Source: CAD feature listing. Evaluate the final solid. Frame: model axes, mm. Give positions to 0.01 mm unless a question says otherwise; leave off trailing zeros. Loops run counter-clockwise (first coordinate to the right, second up) from the corner with the lowest first, then second, coordinate; pieces in that order, holes last. Notation, with made-up numbers: (31.25, -20) -> (54.25, -20) arc R15 ccw to (54.25, -1) -> close; hole circle Ø5 at (-22, -25). An arc over 180 degrees is marked (long way). Put each result on its own line as item: value.
Autodesk Inventor part; units mm, degrees
ref_plane "YZ Plane" through (0, 0, 0) normal (1, 0, 0) x (0, 1, 0)
ref_plane "XZ Plane" through (0, 0, 0) normal (0, 1, 0) x (-1, 0, 0)
ref_plane "XY Plane" through (0, 0, 0) normal (0, 0, 1) x (1, 0, 0)
sketch "Sketch2" plane through (0, 0, 0) normal (0, 1, 0) x (-1, 0, 0)
  line L0 (-179.5, 499.25) -> (179.5, 499.25)
  line L1 (179.5, 499.25) -> (179.5, -499.25)
  line L2 (179.5, -499.25) -> (-179.5, -499.25)
  line L3 (-179.5, -499.25) -> (-179.5, 499.25)
  line L4 (-179.5, 499.25) -> (179.5, -499.25) construction
  line L5 (179.5, 499.25) -> (-179.5, -499.25) construction
  point P0 (0, 0)
  dimension "d2" = 359
  dimension "d3" = 998.5
extrude "Plate1" add sketch "Sketch2" along normal blind 0.5
sketch "Sketch3" plane through (-179, 0.5, -499.25) normal (-1, 0, 0) x (0, -1, 0)
  line L0 (0, 998.5) -> (0, 0)
  line L1 (0, 0) -> (50, 0)
  line L2 (50, 0) -> (50, 998.5)
  line L3 (50, 998.5) -> (0, 998.5)
edge flange "Flange1" height 50 angle 90 thickness 0.5 bend radius 0.5 thickness toward (-1, 0, 0) relief tear relief width 0.5 relief depth 0.25 edges at (-179.5, 0, 0) wall of the first edge with corners at (-179, 0.5, 499.25) (-179, 0.5, -499.25) (-179, -49.5, -499.25) (-179, -49.5, 499.25)
bend "Bend1"
corner "Corner1"
sketch "Sketch6" plane through (179, 0.5, 499.25) normal (1, 0, 0) x (0, 1, 0)
  line L0 (0, -998.5) -> (0, 0)
  line L1 (0, 0) -> (-10, 0)
  line L2 (-10, 0) -> (-10, -998.5)
  line L3 (-10, -998.5) -> (0, -998.5)
edge flange "Flange4" height 10 angle 90 thickness 0.5 bend radius 0.5 thickness toward (1, 0, 0) relief tear relief width 0.5 relief depth 0.25 edges at (179.5, 0, 0) wall of the first edge with corners at (179, 0.5, -499.25) (179, 0.5, 499.25) (179, -9.5, 499.25) (179, -9.5, -499.25)
bend "Bend4"
corner "Corner4"
sketch "Sketch7" plane through (179.5, -9, 499.25) normal (0, -1, 0) x (1, 0, 0)
  line L0 (0, -998.5) -> (0, 0)
  line L1 (0, 0) -> (-10, 0)
  line L2 (-10, 0) -> (-10, -998.5)
  line L3 (-10, -998.5) -> (0, -998.5)
edge flange "Flange5" height 10 angle 90 thickness 0.5 bend radius 0.5 thickness toward (0, -1, 0) relief tear relief width 0.5 relief depth 0.25 edges at (179, -9.5, 0) wall of the first edge with corners at (179.5, -9, -499.25) (179.5, -9, 499.25) (169.5, -9, 499.25) (169.5, -9, -499.25)
bend "Bend5"
corner "Corner5"
equation "\"d3\" = Ancho - 3 * Thickness"
equation "\"d4\" = Thickness"
equation "\"d5\" = BendReliefWidth"
equation "\"d6\" = BendReliefDepth"
equation "\"d7\" = MinimumRemnant"
equation "\"d8\" = TransitionRadius"
equation "\"d11\" = BendRadius"
equation "\"d12\" = CornerReliefSize"
equation "\"d13\" = GapSize"
equation "\"d14\" = JacobiRadiusSize"
equation "\"d35\" = BendReliefWidth"
equation "\"d36\" = BendReliefDepth"
equation "\"d37\" = MinimumRemnant"
equation "\"d38\" = TransitionRadius"
equation "\"d41\" = BendRadius"
equation "\"d42\" = CornerReliefSize"
equation "\"d43\" = GapSize"
equation "\"d44\" = JacobiRadiusSize"
equation "\"d45\" = BendReliefWidth"
equation "\"d46\" = BendReliefDepth"
equation "\"d47\" = MinimumRemnant"
equation "\"d48\" = TransitionRadius"
equation "\"d51\" = BendRadius"
equation "\"d52\" = CornerReliefSize"
equation "\"d53\" = GapSize"
equation "\"d54\" = JacobiRadiusSize"
equation "\"BendRadius\" = Thickness"
equation "\"BendReliefWidth\" = Thickness"
equation "\"BendReliefDepth\" = 0.5 * Thickness"
equation "\"CornerReliefSize\" = 4 * Thickness"
equation "\"MinimumRemnant\" = 2 * Thickness"
equation "\"TransitionRadius\" = BendRadius"
equation "\"JacobiRadiusSize\" = BendRadius"
equation "\"GapSize\" = Thickness"
equation "\"Space5\" = 0"
equation "\"Space6\" = 0"
equation "\"Space7\" = 0"
properties part number "Divisor"
(1) Section A-A on z = 436. Return loops of the section in (x, y).
Calculated:
outline: (-179.5, -49.5) -> (-179, -49.5) -> (-179, -0.5) arc R0.5 cw to (-178.5, 0) -> (178.5, 0) arc R0.5 cw to (179, -0.5) -> (179, -8.5) arc R0.5 cw to (178.5, -9) -> (169.5, -9) -> (169.5, -9.5) -> (178.5, -9.5) arc R1 ccw to (179.5, -8.5) -> (179.5, -0.5) arc R1 ccw to (178.5, 0.5) -> (-178.5, 0.5) arc R1 ccw to (-179.5, -0.5) -> close
(2) Line query: probe 1 along Y at (x, z) = (33, 373); probe 2 along X at (y, z) = (-47, -71.5); probe 3 along X at (y, z) = (-5, 182). Output: solid intervals per line, ascending. Write a range as from..to.
Calculated:
probe 1: y = 0..0.5
probe 2: x = -179.5..-179
probe 3: x = -179.5..-179, 179..179.5
(3) Section C-C on y = -37.5. Return loops of the section in (x, z).
Calculated:
outline: (-179.5, -499.25) -> (-179, -499.25) -> (-179, 499.25) -> (-179.5, 499.25) -> close
(4) Section B-B on x = 115.5. Return loops of the section in (y, z), then the cut area to 3 significant figures.
Calculated:
outline: (0, -499.25) -> (0.5, -499.25) -> (0.5, 499.25) -> (0, 499.25) -> close
area: 499 mm²
(5) First-contact query: P1, Ø24.5, axis at y = -26, z = -238, coming from the +X side; P2, Ø10, axis at x = 77, z = -389, coming from the -Y side; P3, Ø2.5, axis at x = 172.5, z = -224, coming from the -Y side. Flat tips, straight axial feed; report the tip coordinate or a pass-through.
Calculated:
P1: stops at x = -179
P2: stops at y = 0
P3: stops at y = -9.5
(6) Draft query along X for faces 1 (the flat face through (2, 0, 7)), 2 (the flat face through (-179.5, -25, -7)), 3 (the flat face through (2, 0.5, 7)). Return one class per face: released by +X, released by -X, zero draft, split by the parting line, or undercut.
Calculated:
face 1: undercut
face 2: released by -X
face 3: zero draft
